Verification items for the finished model (mm, model axes). Face numbers are marked on the shaded views. Round coordinates to 2 decimals unless told otherwise and drop trailing zeros. Order: outer loops, then holes, each group sorted by start corner. A loop starts at its lowest first (then second) coordinate and runs counter-clockwise, first axis right, second up. Notation, with made-up numbers: (0, -15.5) -> (55, -15.5) arc R10 cw to (55, -7.5) -> close; hole circle Ø7 at (13, 81). An arc over 180 degrees is marked (long way). Return JSON: item names as keys, results as strings. Group by question number.
1) Section check D-D on y = 7.25. Enter the section's corners in (x, z).
2) Scan lines: L1, parallel to Y at x = 2, z = -0.8; L2, parallel to X at y = 12.5, z = 0.85; L3, parallel to Y at x = 22, z = 0.1. Record each from-to range of solid material in increasing order.
3) Depth check by flat-ended pin: pin 1 (1.2 mm diameter, centred on x = 2, y = 18.574, fed in from -Z); pin 2 (3 mm diameter, centred on x = 19.5, y = 10, fed in from +Z); pin 3 (0.8 mm diameter, centred on x = 9.5, z = 0.5, fed in from +Y); pin 4 (1.1 mm diameter, centred on y = 12.5, z = 0.5, fed in from +X). Enter the tip coordinate at first touch or a pass-through.
4) Section check A-A on z = -0.7. Enter the section's corners in (x, y).
5) Section check C-C on x = 7.5. Enter the section's corners in (y, z).
6) Section check B-B on y = 18. Enter the section's corners in (x, z), plus the area to 3 significant figures.
7) Draft check along Y on the marked faces 1 and 2. Enter one of: pulls with the +Y half, pulls with the -Y half, needs draft (parallel to the pull), parting line crosses it, or undercut.
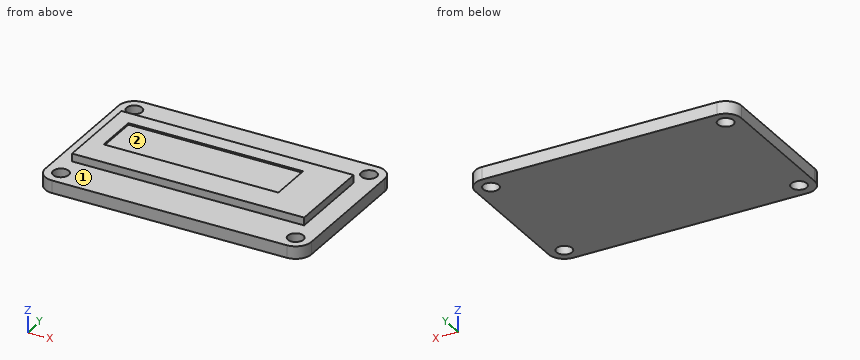
Autodesk Fusion 360 part; units mm, degrees
sketch "Sketch1" plane through (0, 0, 0) normal (0, 0, 1) x (1, 0, 0)
  line L0 (0, 0) -> (34.036, 0)
  line L1 (34.036, 0) -> (34.036, 20.574)
  line L2 (34.036, 20.574) -> (0, 20.574)
  line L3 (0, 20.574) -> (0, 0)
  circle A0 centre (2, 18.574) radius 1
  line L4 (17.018, 20.574) -> (17.018, 0) construction
  line L5 (34.036, 10.287) -> (0, 10.287) construction
  circle A1 centre (32.036, 18.574) radius 1
  circle A2 centre (32.036, 2) radius 1
  circle A3 centre (2, 2) radius 1
  dimension "d1" = 34.036
  dimension "d2" = 20.574
  dimension "d3" = 2
  dimension "d5" = 2
  dimension "d23" = 2
extrude "Extrude1" add sketch "Sketch1" against normal blind 1.6
fillet "Fillet1" radius 2 4 edges at (0, 0, -0.8) (0, 20.574, -0.8) (34.036, 20.574, -0.8) (34.036, 0, -0.8)
sketch "Sketch2" plane through (0, 0, 0) normal (0, 0, 1) x (-1, 0, 0)
  arc A0 (-32.036, 0) -> (-34.036, -2) centre (-32.036, -2) ccw
  line L0 (-34.036, -2) -> (-34.036, -18.574)
  arc A1 (-34.036, -18.574) -> (-32.036, -20.574) centre (-32.036, -18.574) ccw
  line L1 (-32.036, -20.574) -> (-2, -20.574)
  arc A2 (-2, -20.574) -> (0, -18.574) centre (-2, -18.574) ccw
  line L2 (0, -18.574) -> (0, -2)
  arc A3 (0, -2) -> (-2, 0) centre (-2, -2) ccw
  line L3 (-2, 0) -> (-32.036, 0)
  circle A4 centre (-2, -2) radius 1
  circle A5 centre (-32.036, -18.574) radius 1
  circle A6 centre (-2, -18.574) radius 1
  circle A7 centre (-32.036, -2) radius 1
  line L4 (-1.778, -16.074) -> (-31.478, -16.074)
  line L5 (-31.478, -16.074) -> (-31.478, -4.898)
  line L6 (-31.478, -4.898) -> (-1.778, -4.898)
  line L7 (-1.778, -4.898) -> (-1.778, -16.074)
  dimension "d24" = 29.7
  dimension "d25" = 11.176
  dimension "d26" = 4.5
  dimension "d27" = 1.778
extrude "Extrude2" add sketch "Sketch2" along normal blind 1 contours L4 L5 L6 L7
sketch "Sketch3" plane through (0, 0, 1) normal (0, 0, 1) x (-1, 0, 0)
  line L0 (-1.778, -4.898) -> (-31.478, -4.898)
  line L1 (-31.478, -4.898) -> (-31.478, -16.074)
  line L2 (-31.478, -16.074) -> (-1.778, -16.074)
  line L3 (-1.778, -16.074) -> (-1.778, -4.898)
  line L4 (-3.81, -14.042) -> (-26.162, -14.042)
  line L5 (-26.162, -14.042) -> (-26.162, -8.454)
  line L6 (-26.162, -8.454) -> (-3.81, -8.454)
  line L7 (-3.81, -8.454) -> (-3.81, -14.042)
  dimension "d30" = 2.032
  dimension "d31" = 22.352
  dimension "d32" = 5.588
  dimension "d33" = 2.032
extrude "Extrude3" cut sketch "Sketch3" against normal blind 0.2 contours L4 L5 L6 L7
Check result:
{
 "1": {"outline": "(0, -1.6) -> (34.04, -1.6) -> (34.04, 0) -> (31.48, 0) -> (31.48, 1) -> (1.78, 1) -> (1.78, 0) -> (0, 0) -> close"},
 "2": {"L1": "0 to 1, 3 to 17.57, 19.57 to 20.57", "L2": "1.78 to 3.81, 26.16 to 31.48", "L3": "4.9 to 16.07"},
 "3": {"pin 1": "through", "pin 2": "z = 0.8", "pin 3": "y = 16.07", "pin 4": "x = 34.04"},
 "4": {"outline": "(0, 2) arc R2 ccw to (2, 0) -> (32.04, 0) arc R2 ccw to (34.04, 2) -> (34.04, 18.57) arc R2 ccw to (32.04, 20.57) -> (2, 20.57) arc R2 ccw to (0, 18.57) -> close; hole circle Ø2 at (2, 2); hole circle Ø2 at (2, 18.57); hole circle Ø2 at (32.04, 2); hole circle Ø2 at (32.04, 18.57)"},
 "5": {"outline": "(0, -1.6) -> (20.57, -1.6) -> (20.57, 0) -> (16.07, 0) -> (16.07, 1) -> (14.04, 1) -> (14.04, 0.8) -> (8.45, 0.8) -> (8.45, 1) -> (4.9, 1) -> (4.9, 0) -> (0, 0) -> close"},
 "6": {"outline": "(0, -1.6) -> (1.18, -1.6) -> (1.18, 0) -> (0, 0) -> close; (2.82, -1.6) -> (31.22, -1.6) -> (31.22, 0) -> (2.82, 0) -> close; (32.85, -1.6) -> (34.04, -1.6) -> (34.04, 0) -> (32.85, 0) -> close", "area": "49.2 mm^2"},
 "7": {"face 1": "needs draft", "face 2": "undercut"}
}
